Input: dimensioned drawing with shaded views. Units: mm. Origin: part minimum x, y, z. A direction names the side the tool comes from. Coordinates: 2 decimals unless noted, no trailing zeros. Order: outer loops, then holes, each group sorted by start corner. A loop starts at its lowest first (then second) coordinate and runs counter-clockwise, first axis right, second up.
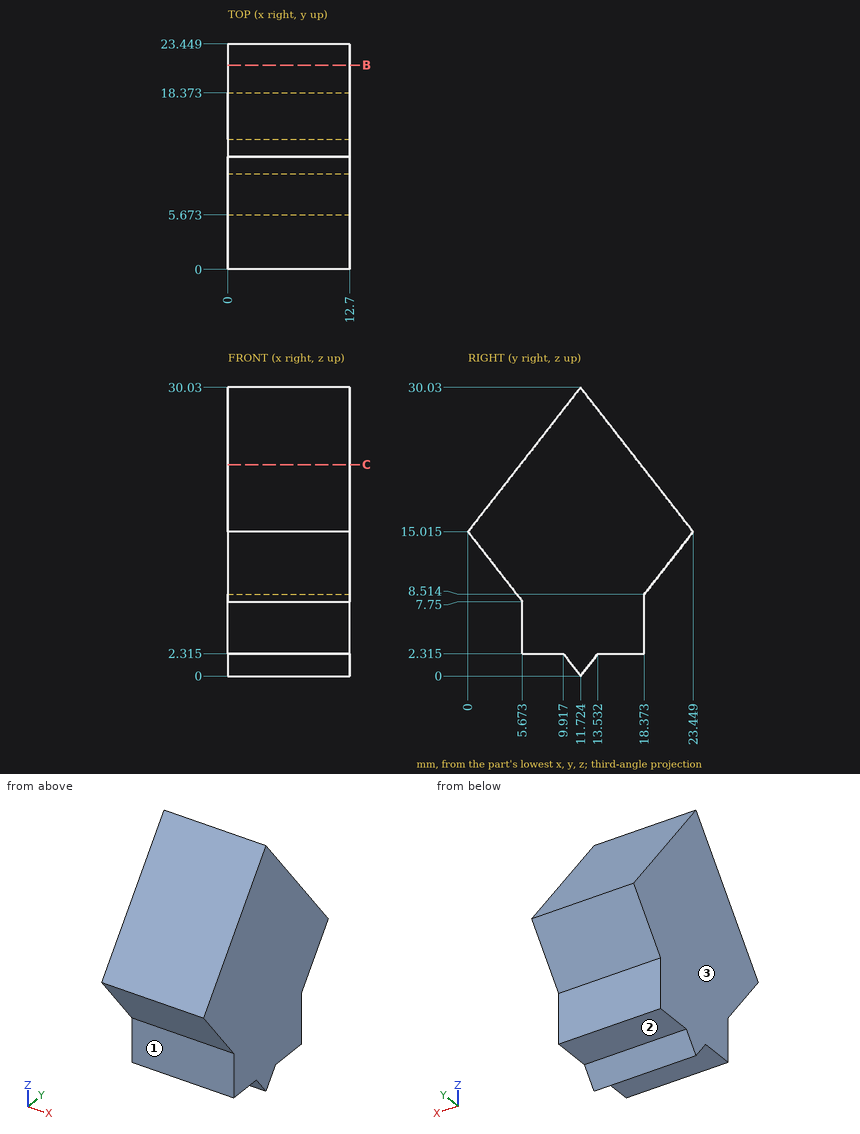
1. Section query C-C on z = 22. Return loops of the section in (x, y) (1 decimal), plus the area to 3 significant figures.
Findings:
outline: (0, 5.5) - (12.7, 5.5) - (12.7, 18) - (0, 18) - close
area: 159 mm2
2. Access query for the marked faces 1, 2 and 3. Directions: +Z, -Z, +X, -X, +Y, -Y. A direction counts if a zero-diameter tool reaches every point of the face in a straight line with its end or side. Return the directions, or none.
Findings:
face 1: -Z, +X, -X, -Y
face 2: -Z, +X, -X, +Y
face 3: +Z, -Z, -X, +Y, -Y
3. Ray query, line 1 (Y direction, x = 6.5, z = 4.5); line 2 (Z direction, x = 11.75, y = 4) (1 decimal); line 3 (Y direction, x = 6.5, z = 10.5) (1 decimal). Return the intervals inside material, ascending.
Findings:
line 1: y = 5.67 to 18.37
line 2: z = 9.9 to 20.1
line 3: y = 3.5 to 19.9
4. Pin query (flat end, axial travel): P1, Ø2.5, axis at x = 8, z = 5, coming from the -Y side; P2, Ø1.3, axis at x = 4, y = 8.5, coming from the -Z side (1 decimal); P3, Ø2, axis at x = 3.5, y = 18.5, coming from the +Z side (1 decimal). Return the tip coordinate at first contact, or that it passes through.
Findings:
P1: stops at y = 5.67
P2: stops at z = 2.3
P3: stops at z = 22.6
5. Section query B-B on y = 21.25. Return loops of the section in (x, z).
Findings:
outline: (0, 12.2) - (12.7, 12.2) - (12.7, 17.83) - (0, 17.83) - close
